Could you check a few things on this model? Use its own coordinates, in mm. A direction names the side the tool comes from. Coordinates: 2 decimals unless noted, no trailing zeros. Order: outer loops, then holes, each group sorted by start corner. A loop starts at its lowest first (then second) coordinate and runs counter-clockwise, first axis right, second up.
```python
from build123d import *

# Parameters (mm, degrees)
BOSS_EXTRUDE1_DEPTH     = 69.85
CUT_EXTRUDE1_DEPTH      = 2.54
CUT_EXTRUDE1_DEPTH_BACK = 105.044993435
SKETCH2_W               = 16.044844987
SKETCH2_H               = 25.145576203
SKETCH2_H_2             = 25.654423797
CUT_EXTRUDE2_DEPTH      = 13.97
FILLET1_R               = 1.016
FILLET2_R               = 2.032
SKETCH4_W               = 34.29
SKETCH4_H               = 15.24
BOSS_EXTRUDE2_DEPTH     = 44.45
FILLET3_R               = 10.16
SKETCH5_R               = 3.5
CUT_EXTRUDE3_DEPTH      = 91.143248047
FILLET4_R               = 7.62


with BuildPart() as part:
    # Sketch1 → Boss-Extrude1 (new body)
    with BuildSketch(Plane.XY):
        with BuildLine():
            Line((3.429, -21.315957849), (3.429, -24.871957849))
            Line((3.429, -24.871957849), (0, -24.871957849))
            Line((0, -24.871957849), (-25.4, -24.871957849))
            Line((-25.4, -24.871957849), (-25.4, 47.724146141))
            Line((-25.4, 47.724146141), (0, 48.429639909))
            Line((0, 48.429639909), (3.429, 48.429639909))
            Line((3.429, 48.429639909), (3.429, 44.873639909))
            ThreePointArc((3.429, 44.873639909), (-11.15, 34.264), (3.429, 23.654360091))
            Line((3.429, 23.654360091), (3.429, 21.315957849))
            ThreePointArc((3.429, 21.315957849), (-21.59, 0), (3.429, -21.315957849))
        make_face()
    extrude(amount=-BOSS_EXTRUDE1_DEPTH)

    # Sketch2 → Cut-Extrude1 (cut, two sides: drawn at the far end of the back side and taken through both)
    with BuildSketch(Plane(origin=(-1.344113023, 48.392306706, 0), x_dir=(0.9996144881434057, 0.027764637469221053, 0), z_dir=(-0.027764637469221053, 0.9996144881434057, 0)).offset(-CUT_EXTRUDE1_DEPTH_BACK)):
        with Locations((2.634731969, 50.927211899)):
            Rectangle(SKETCH2_W, SKETCH2_H)
        with Locations((2.634731969, 19.177211899)):
            Rectangle(SKETCH2_W, SKETCH2_H_2)
    extrude(amount=CUT_EXTRUDE1_DEPTH + CUT_EXTRUDE1_DEPTH_BACK, mode=Mode.SUBTRACT)

    # Sketch3 → Cut-Extrude2 (cut)
    with BuildSketch(Plane.XZ.offset(24.871957849)):
        Polygon((-4.69894113, -6.35), (-14.85894113, -6.35), (-14.85894113, -32.004423797), (-7.683449997, -32.004423797), (-4.37926474, -32.004423797), (-4.37926474, -6.35), align=None)
        Polygon((-4.69894113, -38.354423797), (-14.85894113, -38.354423797), (-14.85894113, -63.5), (-7.683449997, -63.5), (-2.422701427, -63.5), (-2.422701427, -38.354423797), align=None)
    extrude(amount=-CUT_EXTRUDE2_DEPTH, mode=Mode.SUBTRACT)

    # Fillet1
    # the kernel refuses this fillet: 1.016 mm, written as the material it takes off along each edge
    with BuildSketch(Plane(origin=(3.429, -21.315957849, -60.597776235), x_dir=(-0.9911390490997786, -0.13282840565777682, 0), z_dir=(0, 0, -1)), Plane(origin=(3.429, -21.315957849, -29.102200032), x_dir=(-0.9911390490997786, -0.13282840565777682, 0), z_dir=(0, 0, -1))) as fillet1_piece_1:
        with BuildLine():
            CenterArc((1.161196376, -1.015649261), FILLET1_R, 91.505550469, 96.127515329)
            Line((0.154199102, -1.150602921), (0, 0))
            ThreePointArc((0, 0), (0.567251103, -0.007453204), (1.134502207, 0))
        make_face()
    extrude(amount=12.15444753, mode=Mode.SUBTRACT)
    with BuildSketch(Plane(origin=(3.429, 44.873639909, -60.213343849), x_dir=(-0.967377188342964, 0.25334043394938266, 0), z_dir=(0, 0, -1)), Plane(origin=(3.429, 44.873639909, -28.717767646), x_dir=(-0.967377188342964, 0.25334043394938266, 0), z_dir=(0, 0, -1)), Plane(origin=(3.429, 44.873639909, 3.286656151), x_dir=(-0.967377188342964, 0.25334043394938266, 0), z_dir=(0, 0, -1))) as fillet1_piece_2:
        with BuildLine():
            CenterArc((1.315912382, 1.014380594), FILLET1_R, 165.324729703, 101.43988218)
            Line((0.333057158, 1.271774475), (0, 0))
            ThreePointArc((0, 0), (0.6292856, 0.017772027), (1.2585712, 0))
        make_face()
    extrude(amount=12.923312302, mode=Mode.SUBTRACT)
    with BuildSketch(Plane(origin=(3.429, 23.654360091, -60.213343849), x_dir=(-0.9673771883429638, -0.2533404339493828, 0), z_dir=(0, 0, -1)), Plane(origin=(3.429, 23.654360091, -28.717767646), x_dir=(-0.9673771883429638, -0.2533404339493828, 0), z_dir=(0, 0, -1)), Plane(origin=(3.429, 23.654360091, 3.286656151), x_dir=(-0.9673771883429638, -0.2533404339493828, 0), z_dir=(0, 0, -1))) as fillet1_piece_3:
        with BuildLine():
            CenterArc((1.315912382, -1.014380594), FILLET1_R, 93.235388117, 101.43988218)
            Line((0.333057158, -1.271774475), (0, 0))
            ThreePointArc((0, 0), (0.6292856, -0.017772027), (1.2585712, 0))
        make_face()
    extrude(amount=12.923312302, mode=Mode.SUBTRACT)
    with BuildSketch(Plane(origin=(3.429, 21.315957849, -60.597776235), x_dir=(-0.9911390490997777, 0.13282840565778328, 0), z_dir=(0, 0, -1)), Plane(origin=(3.429, 21.315957849, -29.102200032), x_dir=(-0.9911390490997777, 0.13282840565778328, 0), z_dir=(0, 0, -1)), Plane(origin=(3.429, 21.315957849, 2.902223765), x_dir=(-0.9911390490997777, 0.13282840565778328, 0), z_dir=(0, 0, -1))) as fillet1_piece_4:
        with BuildLine():
            CenterArc((1.161196376, 1.015649261), FILLET1_R, 172.366934203, 96.127515328)
            Line((0.154199102, 1.150602921), (0, 0))
            ThreePointArc((0, 0), (0.567251103, 0.007453204), (1.134502207, 0))
        make_face()
    extrude(amount=12.15444753, mode=Mode.SUBTRACT)
    with BuildSketch(Plane(origin=(3.429, -21.315957849, 2.902223765), x_dir=(0, -1, 0), z_dir=(0, 0, -1))) as fillet1_piece_5:
        with BuildLine():
            CenterArc((1.160889506, 1.016), FILLET1_R, 173.872484672, 96.127515328)
            ThreePointArc((0.150694119, 1.124449438), (0.082734222, 0.561234722), (0, 0))
            Line((0, 0), (1.160889506, 0))
        make_face()
    extrude(amount=12.15444753, mode=Mode.SUBTRACT)

    # Fillet2
    fillet2_edges = [part.edges().sort_by_distance(p)[0] for p in [
        (-14.85894113, -20.267644911, -6.35),
        (-14.85894113, -20.267644911, -32.004423797),
        (-14.85894113, -20.267644911, -38.354423797),
        (-14.85894113, -20.267644911, -63.5),
        (-6.023991911, 22.834048029, -63.5),
        (-6.660489458, 45.749966547, -63.5),
        (-6.660489458, 45.749966547, -38.354423797),
        (-6.023991911, 22.834048029, -38.354423797),
        (-6.023991911, 22.834048029, -32.004423797),
        (-6.660489458, 45.749966547, -32.004423797),
        (-6.660489458, 45.749966547, -6.35),
        (-6.023991911, 22.834048029, -6.35),
    ]]
    fillet(fillet2_edges, radius=FILLET2_R)

    # Sketch4 → Boss-Extrude2 (add)
    with BuildSketch(Plane.ZY.offset(25.4)):
        with Locations((17.145, 18.514146141)):
            Rectangle(SKETCH4_W, SKETCH4_H)
    extrude(amount=-BOSS_EXTRUDE2_DEPTH)

    # Fillet3
    fillet3_edges = [part.edges().sort_by_distance(p)[0] for p in [
        (19.05, 18.514146141, 0),
        (19.05, 18.514146141, 34.29),
    ]]
    fillet(fillet3_edges, radius=FILLET3_R)

    # Sketch5 → Cut-Extrude3 (cut, through all)
    with BuildSketch(Plane(origin=(0, 26.134146141, 0), x_dir=(1, 0, 0), z_dir=(0, 1, 0))):
        with Locations(Location((10.91, -24.892, 0), (0, 0, 270))):
            Circle(SKETCH5_R)
        with Locations(Location((-15.98, -25, 0), (0, 0, 270))):
            Circle(SKETCH5_R)
    extrude(amount=-CUT_EXTRUDE3_DEPTH, mode=Mode.SUBTRACT)

    # Fillet4
    fillet4_edges = [part.edges().sort_by_distance(p)[0] for p in [
        (-25.4, -24.871957849, -34.925),
        (-25.4, 47.724146141, -34.925),
    ]]
    fillet(fillet4_edges, radius=FILLET4_R)


solid = part.part
```
Item 1: Suppose I cut it at B-B (z = -48.5). List the corners of the cut face in (x, y) for me, and give its area (3 significant figures).
Item 2: Suppose I cut it at C-C (x = -9). List the corners of the cut face in (y, z) for me, and give its area (3 significant figures).
Item 3: Which directions (+Z, -Z, +X, -X, +Y, -Y) give clear straight access to the entire face, cutting with the end or side of a thin tool? Please do faces 1 (the face through (-3, 10.894, 17)), 2 (the face through (-7, -23, -6.35)), 3 (the face through (-5.446, 22.879, -62.889)).
Item 4: Suppose I cut it at A-A (x = 13). List the corners of the cut face in (y, z) for me.
Item 5: Suppose I cut it at D-D (x = -15.98). List the corners of the cut face in (y, z) for me.
Item 6: Thinking about a two-plate mould opening in Z: for faces 4 (the face through (-14.25, -20.2, -6.93)), 5 (the face through (2, 48.43, -67)), 6 (the face through (-17, 20, -69.85)), which applies, +Z half, -Z half, draft (parallel to the pull), parting line (faces both ways), or undercut?
Item 7: I need wall thicknesses on line 1 (Z direction, x = -13, y = -19.5); line 2 (X direction, y = 22, z = 25); line 3 (Y direction, x = -1, z = -64.5). Which ranges of each line are inside material? Lowest first, please.
Item 8: For pin 1 Ø10 at (x, z) = (-20.5, -2) entering from -Y; pin 2 Ø2.5 at (y, z) = (-24, -36.5) entering from +X; pin 3 Ø8 at (x, z) = (-18, 21) entering from -Y; pin 4 Ø4 at (x, y) = (-5, -19.5) entering from +Z, each with a flat end and sliding along its axis, tell me the tip position at first contact or that it passes through.
Geometry results:
1. outline: (-25.4, -17.25) arc R7.62 ccw to (-17.78, -24.87) - (-14.86, -24.87) - (-14.86, -15.66) arc R21.59 cw to (-5.97, 20.75) - (-6.08, 24.92) arc R11.15 cw to (-6.59, 43.26) - (-6.73, 48.24) - (-17.99, 47.93) arc R7.62 ccw to (-25.4, 40.31) - close
1. area: 787 mm2
2. outline: (-24.87, -69.85) - (-19.62, -69.85) - (-19.62, -63.5) - (-24.87, -63.5) - close; (-24.87, -38.35) - (-19.62, -38.35) - (-19.62, -32) - (-24.87, -32) - close; (-24.87, -6.35) - (-19.62, -6.35) - (-19.62, 0) - (-24.87, 0) - close; (10.89, 0) - (19.62, 0) - (19.62, -69.85) - (27.68, -69.85) - (27.68, 0) - (26.13, 0) - (26.13, 34.29) - (10.89, 34.29) - close; (40.85, -69.85) - (48.18, -69.85) - (48.18, 0) - (40.85, 0) - close
2. area: 1,700 mm2
3. face 1: +Z, +X, -X, -Y
3. face 2: +X, -Y
3. face 3: +X, +Y
4. outline: (10.89, 0.87) - (26.13, 0.87) - (26.13, 22.08) - (10.89, 22.08) - close; (10.89, 27.7) - (26.13, 27.7) - (26.13, 33.42) - (10.89, 33.42) - close
5. outline: (-24.87, -69.85) - (-14.52, -69.85) - (-14.52, 0) - (-24.87, 0) - close; (10.89, 0) - (14.52, 0) - (14.52, -69.85) - (47.99, -69.85) - (47.99, 0) - (26.13, 0) - (26.13, 21.5) - (10.89, 21.5) - close; (10.89, 28.5) - (26.13, 28.5) - (26.13, 34.29) - (10.89, 34.29) - close
6. face 4: undercut
6. face 5: draft
6. face 6: -Z half
7. line 1: z = -69.85 to -63.49, -38.36 to -32, -6.36 to 0
7. line 2: x = -25.4 to -19.48, -12.48 to 7.41, 14.41 to 19.01
7. line 3: y = -24.87 to -21.57, 21.57 to 23.16, 45.37 to 48.4
8. pin 1: stops at y = -24.87
8. pin 2: stops at x = 3.43
8. pin 3: stops at y = 10.89
8. pin 4: stops at z = 0
